Verification items for this drawing (mm, ordinates from the low corner). Give positions to 0.01 mm unless a question says otherwise; leave off trailing zeros. Loops run counter-clockwise (first coordinate to the right, second up) from the corner with the lowest first, then second, coordinate; pieces in that order, holes last. Notation, with made-up numbers: M 10.5,70.25 L 47.5,70.25 A20 ccw 47.5,103.25 Z; hole C -6.75,39.5 d9. An arc over 180 degrees is marked long. Use one line per item in the form item = value.
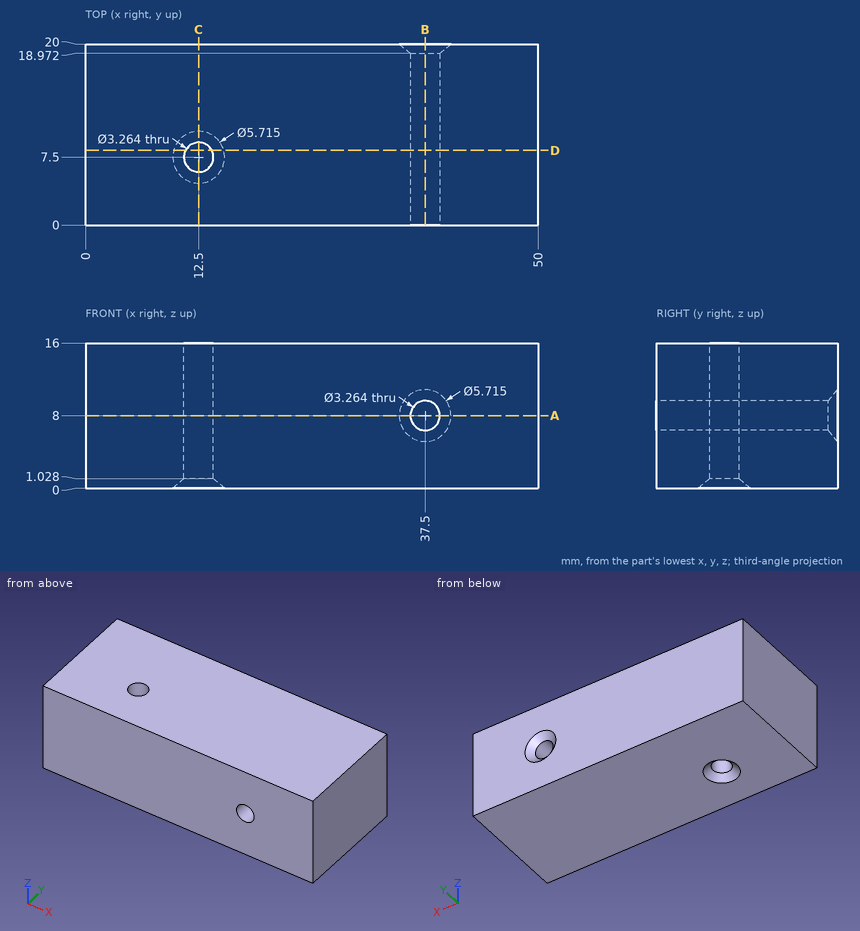
1) Scan lines: line 1 (Z direction, x = 37.5, y = 13.5); line 2 (Y direction, x = 12.5, z = 7.25); line 3 (X direction, y = 14, z = 8). Record each from-to range of solid material in increasing order.
Evaluation:
line_1 = 0 to 6.37, 9.63 to 16
line_2 = 0 to 5.87, 9.13 to 20
line_3 = 0 to 35.87, 39.13 to 50
2) Section check B-B (x = 37.5). Record the cut outline in (y, z).
Evaluation:
outline = M 0,0 L 20,0 L 20,5.14 L 18.97,6.37 L 0,6.37 Z; M 0,9.63 L 18.97,9.63 L 20,10.86 L 20,16 L 0,16 Z
3) Section check D-D (y = 8.25). State how many separate pieces and enclosed holes the cut face has, then the cut area to 3 significant figures.
Evaluation:
separate_pieces = 2
enclosed_holes = 1
area = 744 mm^2
4) Section check C-C (x = 12.5). Record the cut outline in (y, z).
Evaluation:
outline = M 0,0 L 4.64,0 L 5.87,1.03 L 5.87,16 L 0,16 Z; M 9.13,1.03 L 10.36,0 L 20,0 L 20,16 L 9.13,16 Z
5) Section check A-A (z = 8). Record the cut outline in (x, y), then the cut area to 3 significant figures.
Evaluation:
outline = M 0,0 L 35.87,0 L 35.87,18.97 L 34.64,20 L 0,20 Z; M 39.13,0 L 50,0 L 50,20 L 40.36,20 L 39.13,18.97 Z; hole C 12.5,7.5 d3.26
area = 925 mm^2
6) Depth check by flat-ended pin: pin 1 Ø4 at (x, y) = (12.5, 7.5) entering from -Z. Enter the tip coordinate at first touch or a pass-through.
Evaluation:
pin_1 = 0.72
